The model under review builds one solid part; all positions refer to its coordinate system, in mm. A direction names the side the tool comes from. Give positions to 0.01 mm unless a question says otherwise; leave off trailing zeros. Write each loop counter-clockwise with the first axis right and the second up, starting at its lowest first coordinate (ties: lowest second). Pieces come first, ordered by that corner, then holes. Notation, with made-up numbers: (-35, 30.5) - (-12, 30.5) arc R33 cw to (-12, 66.5) - close; hole circle Ø1 at (-27, 44). An arc over 180 degrees is marked (long way). Write item = value, one per line.
```python
from build123d import *
from build123d.topology import SkipClean

# Parameters (mm, degrees)
EXTRUDE_1_DEPTH     = 1
SKETCH_3_R          = 9.7
SKETCH_3_R_2        = 1.15
CUT_EXTRUDE_1_DEPTH = 60.104137335
SKETCH_4_R          = 12.2
SKETCH_4_R_2        = 10.5
EXTRUDE_2_DEPTH     = 4
CUT_EXTRUDE_2_DEPTH = 60.230896077


with BuildPart() as part:
    # 草图2 → 凸台-拉伸1 (new body)
    with BuildSketch(Plane.XY):
        with BuildLine():
            Line((-47.999535461, 22.106463733), (-48.193482209, -0.117632256))
            ThreePointArc((-48.193482209, -0.117632256), (-44.33750525, -9.426784127), (-34.962475131, -13.1197067))
            Line((-34.962475131, -13.1197067), (0.319358769, -12.195819365))
            ThreePointArc((0.319358769, -12.195819365), (11.588061422, 3.815341724), (-6.988562084, 10))
            Line((-6.988562084, 10), (-17.408374558, 10))
            ThreePointArc((-17.408374558, 10), (-18.744566439, 10.181847734), (-19.983564933, 10.714163496))
            Line((-19.983564933, 10.714163496), (-22.14712826, 12.014163496))
            ThreePointArc((-22.14712826, 12.014163496), (-24.275653905, 14.604401107), (-24.289397802, 17.956976744))
            ThreePointArc((-24.289397802, 17.956976744), (-33.696855253, 34.017353376), (-47.999535461, 22.106463733))
        make_face()
    extrude(amount=-EXTRUDE_1_DEPTH)

    # 草图3 → 切除-拉伸1 (cut, through all)
    with BuildSketch(Plane.XY):
        with BuildLine():
            ThreePointArc((-18, 8.5), (-19.060660172, 8.060660172), (-19.5, 7))
            Line((-19.5, 7), (-19.5, -7))
            ThreePointArc((-19.5, -7), (-19.060660172, -8.060660172), (-18, -8.5))
            Line((-18, -8.5), (-11.144505373, -8.5))
            ThreePointArc((-11.144505373, -8.5), (-10.131929949, -7.895152283), (-10.184491801, -6.716853933))
            ThreePointArc((-10.184491801, -6.716853933), (-12.2, 0), (-10.184491801, 6.716853933))
            ThreePointArc((-10.184491801, 6.716853933), (-10.131929949, 7.895152283), (-11.144505373, 8.5))
            Line((-11.144505373, 8.5), (-18, 8.5))
        make_face()
        with BuildLine():
            ThreePointArc((-41.944525547, 11.460322311), (-43.44725776, 11.465077783), (-44.2, 10.1644603))
            Line((-44.2, 10.1644603), (-44.2, 4.626978026))
            ThreePointArc((-44.2, 4.626978026), (-43.538789355, 3.383421667), (-42.13809011, 3.236202244))
            Line((-42.13809011, 3.236202244), (-28.13809011, 8.892569405))
            ThreePointArc((-28.13809011, 8.892569405), (-27.358855493, 10.955157224), (-29.477372263, 11.566190605))
            ThreePointArc((-29.477372263, 11.566190605), (-35.696404047, 9.800439849), (-41.944525547, 11.460322311))
        make_face()
        with BuildLine():
            Line((-26.75, -4.5), (-37.75, -4.5))
            ThreePointArc((-37.75, -4.5), (-38.457106781, -4.792893219), (-38.75, -5.5))
            Line((-38.75, -5.5), (-38.75, -8.5))
            ThreePointArc((-38.75, -8.5), (-38.457106781, -9.207106781), (-37.75, -9.5))
            Line((-37.75, -9.5), (-26.75, -9.5))
            ThreePointArc((-26.75, -9.5), (-26.042893219, -9.207106781), (-25.75, -8.5))
            Line((-25.75, -8.5), (-25.75, -5.5))
            ThreePointArc((-25.75, -5.5), (-26.042893219, -4.792893219), (-26.75, -4.5))
        make_face()
        Circle(SKETCH_3_R)
        with Locations((-35.8, 22)):
            Circle(SKETCH_3_R)
        with Locations((-43.8, -0.5)):
            Circle(SKETCH_3_R_2)
        with Locations((-27.8, -0.5)):
            Circle(SKETCH_3_R_2)
        with Locations((-22.5, 8)):
            Circle(SKETCH_3_R_2)
        with Locations((-22.5, -8)):
            Circle(SKETCH_3_R_2)
    extrude(amount=-CUT_EXTRUDE_1_DEPTH, mode=Mode.SUBTRACT)

    # 草图4 → 凸台-拉伸2 (add)
    # profile 1 of 2: a face of its own
    with BuildSketch(Plane.XY.offset(-1)):
        with Locations((-35.8, 22)):
            Circle(SKETCH_4_R)
        with Locations((-35.8, 22)):
            Circle(SKETCH_4_R_2, mode=Mode.SUBTRACT)
    # profile 2 of 2: a face of its own
    with BuildSketch(Plane.XY.offset(-1)):
        Circle(SKETCH_4_R)
        Circle(SKETCH_4_R_2, mode=Mode.SUBTRACT)
    extrude(amount=-EXTRUDE_2_DEPTH)

    # 草图6 → 切除-拉伸2 (cut, through all)
    with SkipClean():  # the faces are left unmerged after this step: merging them gives an invalid solid
        with BuildSketch(Plane(origin=(0, 0, -1), x_dir=(-1, 0, 0), z_dir=(0, 0, -1))):
            with BuildLine():
                Line((47.999535461, 22.106463733), (48.193482209, -0.117632256))
                ThreePointArc((48.193482209, -0.117632256), (44.33750525, -9.426784127), (34.962475131, -13.1197067))
                Line((34.962475131, -13.1197067), (-0.319358769, -12.195819365))
                ThreePointArc((-0.319358769, -12.195819365), (2.156225392, -12.007942874), (4.542515187, -11.322789222))
                Line((4.542515187, -11.322789222), (34.988652079, -12.120049375))
                ThreePointArc((34.988652079, -12.120049375), (43.636595985, -8.713533678), (47.193520286, -0.126358792))
                Line((47.193520286, -0.126358792), (47.041786885, 17.26056674))
                ThreePointArc((47.041786885, 17.26056674), (47.768482684, 19.634535512), (47.999535461, 22.106463733))
            make_face()
        extrude(amount=-CUT_EXTRUDE_2_DEPTH, mode=Mode.SUBTRACT)


solid = part.part
```
1. Take a section at B-B on z = -2.95. Give the boundary of the cut face in (x, y), and give its area (3 significant figures).
Findings below:
outline = circle Ø24.4 at (-35.8, 22); circle Ø24.4 at (0, 0); hole circle Ø21 at (-35.8, 22); hole circle Ø21 at (0, 0)
area = 242 mm²
2. Machinability: for faces 3 (the cylindrical face through (-43.428, 11.476, -0.493)), 4 (the flat face through (-21.05, 11.355, -0.493)), 5 (the cylindrical face through (10, 3.2, -3)), which of the approach directions +Z, -Z, +X, -X, +Y, -Y give a long, thin tool a straight path to every point of the face, cutting with its end or side? Answer none if there is none.
Findings below:
face_3 = +Z, -Z
face_4 = +Z, -Z, +Y
face_5 = -Z
3. Take a section at C-C on x = -8.5. Give the boundary of the cut face in (y, z).
Findings below:
outline = (-11.43, -1) - (-8.75, -1) - (-8.75, -5) - (-6.16, -5) - (-6.16, -1) - (-4.67, -1) - (-4.67, 0) - (-11.43, 0) - close; (4.67, -1) - (6.16, -1) - (6.16, -5) - (8.75, -5) - (8.75, -1) - (10, -1) - (10, 0) - (4.67, 0) - close
4. Draft analysis for pull direction X (two halves, no side actions). For faces 1 (the flat face through (-30, 31, -5)), 2 (the cylindrical face through (-27.34, 10.92, -0.49)), state which applies: +X half, -X half, draft (parallel to the pull), parting line (faces both ways), or undercut.
Findings below:
face_1 = draft
face_2 = undercut
5. Insertion check: P1, Ø0.5, axis at x = -14, z = -0.5, coming from the +Y side; P2, Ø0.8, axis at y = 8, z = -0.5, coming from the +X side; P3, Ø1.8, axis at x = -28.7, y = 10.28, coming from the -Z side; P4, Ø1.1, axis at x = -29.5, z = -0.5, coming from the +Y side. Each pin has a flat end and moves straight along its axis. Give the tip position at first contact, or say it passes through.
Findings below:
P1 = 10
P2 = 9.54
P3 = through
P4 = 32.76
6. Take a section at A-A on y = -2.5. Give the boundary of the cut face in (x, z).
Findings below:
outline = (-46.98, -1) - (-19.5, -1) - (-19.5, 0) - (-46.98, 0) - close; (-11.94, -5) - (-10.2, -5) - (-10.2, -1) - (-9.37, -1) - (-9.37, 0) - (-11.94, 0) - close; (9.37, -1) - (10.2, -1) - (10.2, -5) - (11.94, -5) - (11.94, 0) - (9.37, 0) - close
7. Take a section at D-D on y = 16. Give the boundary of the cut face in (x, z), and give its area (3 significant figures).
Findings below:
outline = (-47.05, -1) - (-46.42, -1) - (-46.42, -5) - (-44.42, -5) - (-44.42, -1) - (-43.42, -1) - (-43.42, 0) - (-47.05, 0) - close; (-28.18, -1) - (-27.18, -1) - (-27.18, -5) - (-25.18, -5) - (-25.18, -1) - (-24.56, -1) - (-24.56, 0) - (-28.18, 0) - close
area = 23.3 mm²
8. For line 1 (X direction, y = -7.5, z = -0.4); line 2 (Y direction, x = -0.5, z = -4.8); line 3 (Y direction, x = -27.8, z = -0.3), list the stretches that pass through material, from the lowest coordinate up. Write a range as from..to.
Findings below:
line_1 = -44.71..-38.75, -25.75..-23.54, -21.46..-19.41, -10..-6.15, 6.15..9.62
line_2 = -12.19..-10.49, 10.49..12.19
line_3 = -11.93..-9.5, -4.5..-1.65, 0.65..9.08, 11.48..16.51, 27.49..31.21
